Read the model definition and answer for the solid it produces. Units are mm, in the model's axes. A direction names the side the tool comes from. Coordinates: 2 decimals unless noted, no trailing zeros. Loops run counter-clockwise (first coordinate to the right, second up) from the corner with the lowest first, then second, coordinate; pieces in that order, holes last. Notation, with made-up numbers: M -14.5,87 L 3.5,87 A23 ccw 3.5,104 Z; hole C 78,-12.5 d3. An arc over 180 degrees is marked long. One line per item, written item: value. Start each with the question number.
```python
from build123d import *

# Parameters (mm, degrees)
SKETCH1_W           = 22
SKETCH1_H           = 82.75
SKETCH1_R           = 3.1
BOSS_EXTRUDE1_DEPTH = 30
SKETCH2_W           = 22
SKETCH2_H           = 82.75
BOSS_EXTRUDE2_DEPTH = 5
SKETCH3_W           = 16
SKETCH3_H           = 35
SKETCH3_R           = 3.1
SKETCH3_W_2         = 22
SKETCH3_H_2         = 14
BOSS_EXTRUDE3_DEPTH = 5
BOSS_EXTRUDE5_START = 15
SKETCH5_R           = 3.1
BOSS_EXTRUDE5_DEPTH = 15


with BuildPart() as part:
    # Sketch1 → Boss-Extrude1 (new body)
    with BuildSketch(Plane.XY):
        with Locations((0, 7.844654309)):
            Rectangle(SKETCH1_W, SKETCH1_H)
        with Locations((0, 35.719654309)):
            Circle(SKETCH1_R, mode=Mode.SUBTRACT)
        with Locations((0, 7.719654309)):
            Circle(SKETCH1_R, mode=Mode.SUBTRACT)
    extrude(amount=BOSS_EXTRUDE1_DEPTH)

    # Sketch2 → Boss-Extrude2 (add)
    with BuildSketch(Plane.XY.offset(30)):
        with Locations((0, 7.844654309)):
            Rectangle(SKETCH2_W, SKETCH2_H)
    extrude(amount=BOSS_EXTRUDE2_DEPTH)

    # Sketch3 → Boss-Extrude3 (add)
    # profile 1 of 2: a face of its own
    with BuildSketch(Plane.XZ.offset(33.530345691)):
        with Locations((-19, 17.5)):
            Rectangle(SKETCH3_W, SKETCH3_H)
        with Locations(Location((-19, 26, 0), (0, 0, 270))):
            Circle(SKETCH3_R, mode=Mode.SUBTRACT)
        with Locations(Location((-19, 9, 0), (0, 0, 270))):
            Circle(SKETCH3_R, mode=Mode.SUBTRACT)
    # profile 2 of 2: a face of its own
    with BuildSketch(Plane.XZ.offset(33.530345691)):
        with Locations((0, -7)):
            Rectangle(SKETCH3_W_2, SKETCH3_H_2)
        with Locations(Location((0, -7, 0), (0, 0, 270))):
            Circle(SKETCH3_R, mode=Mode.SUBTRACT)
    extrude(amount=-BOSS_EXTRUDE3_DEPTH)

    # Sketch5 → Boss-Extrude5 (add)
    with BuildSketch(Plane(origin=(0, 0, 30), x_dir=(-1, 0, 0), z_dir=(0, 0, -1)).offset(BOSS_EXTRUDE5_START)):
        with Locations((0, 7.719654309)):
            Circle(SKETCH5_R)
        with Locations((0, 35.719654309)):
            Circle(SKETCH5_R)
    extrude(amount=-BOSS_EXTRUDE5_DEPTH)


solid = part.part
```
1) Flat-ended cylindrical pins translate along their axes: pin 1 (8 mm diameter, centred on x = -22, z = 28, fed in from +Y); pin 2 (8 mm diameter, centred on x = -17.5, y = -13.5, fed in from +Z); pin 3 (10.5 mm diameter, centred on y = 24.5, z = 12, fed in from -X); pin 4 (1.9 mm diameter, centred on x = -1, y = 34.5, fed in from -Z). Find the tip coordinate at first contact, or state that the pin passes through.
2) Section A-A (x = 0) is taken. Determine the outline of the cut face in (y, z), then the cut area to 3 significant figures.
3) Section D-D (z = 9) is taken. Determine the outline of the cut face in (x, y).
4) Section C-C (x = -19) is taken. Determine the outline of the cut face in (y, z), then the cut area to 3 significant figures.
5) A tool of negligible diameter and unlimited length cuts with its end or side. For faces 5 (the face through (-19, -28.53, 18)), 6 (the face through (0, 11, 0)), 7 (the face through (0, 36, 15)), 8 (the face through (-19, -31, 0)), 9 (the face through (-4, -33.53, 16)), from which of +Z, -Z, +X, -X, +Y, -Y can it reach the whole face along a straight path? Write none if from no direction.
6) Section B-B (z = 26) is taken. Determine the outline of the cut face in (x, y).
7) For a pull along X with two mould halves and no side action, classify faces 1 (the face through (0, 49.22, 17)), 2 (the face through (-0.7, 4.7, 7.4)), 3 (the face through (0, 8, 15)), 4 (the face through (11, 7, 16)) as released by +X, released by -X, zero draft, split by the parting line, or undercut.
8) Consider line 1 along Y through (x, z) = (0, 3.5); line 2 along X through (y, z) = (-30.5, 26); line 3 along X through (y, z) = (-32, -7). Determine where each line is inside the solid, lowest interval first.
Results found:
1. pin 1: stops at y = -28.53
1. pin 2: passes through
1. pin 3: stops at x = -11
1. pin 4: stops at z = 15
2. outline: M -33.53,-14 L -28.53,-14 L -28.53,-10.1 L -33.53,-10.1 Z; M -33.53,-3.9 L -28.53,-3.9 L -28.53,0 L 4.62,0 L 4.62,15 L 10.82,15 L 10.82,0 L 32.62,0 L 32.62,15 L 38.82,15 L 38.82,0 L 49.22,0 L 49.22,35 L -33.53,35 Z
2. area: 2,750 mm²
3. outline: M -27,-33.53 L -22.1,-33.53 L -22.1,-28.53 L -27,-28.53 Z; M -15.9,-33.53 L 11,-33.53 L 11,49.22 L -11,49.22 L -11,-28.53 L -15.9,-28.53 Z; hole C 0,7.72 d6.2; hole C 0,35.72 d6.2
4. outline: M -33.53,0 L -28.53,0 L -28.53,5.9 L -33.53,5.9 Z; M -33.53,12.1 L -28.53,12.1 L -28.53,22.9 L -33.53,22.9 Z; M -33.53,29.1 L -28.53,29.1 L -28.53,35 L -33.53,35 Z
4. area: 113 mm²
5. face 5: +Z, -Z, -X, +Y
5. face 6: -Z, +X, -X, +Y
5. face 7: -Z
5. face 8: -Z, -X, +Y, -Y
5. face 9: +Z, -Z, +X, -X, -Y
6. outline: M -27,-33.53 L -22.1,-33.53 L -22.1,-28.53 L -27,-28.53 Z; M -15.9,-33.53 L 11,-33.53 L 11,49.22 L -11,49.22 L -11,-28.53 L -15.9,-28.53 Z
7. face 1: zero draft
7. face 2: undercut
7. face 3: undercut
7. face 4: released by +X
8. line 1: y = -33.53 to 4.62, 10.82 to 32.62, 38.82 to 49.22
8. line 2: x = -27 to -22.1, -15.9 to 11
8. line 3: x = -11 to -3.1, 3.1 to 11
